Source: three-view drawing plus pictorial views. Frame: mm from the lowest corner of the part. Give positions to 0.01 mm unless a question says otherwise; leave off trailing zeros. Order: outer loops, then holes, each group sorted by start corner. A loop starts at its lowest first (then second) coordinate and runs counter-clockwise, first axis right, second up. Notation, with made-up numbers: (-35, -9.5) -> (-23, -9.5) arc R24 cw to (-23, 26.5) -> close; hole circle Ø10 at (-27, 15.25). An arc over 180 degrees is marked (long way). One line per question, with ' | ' between items.
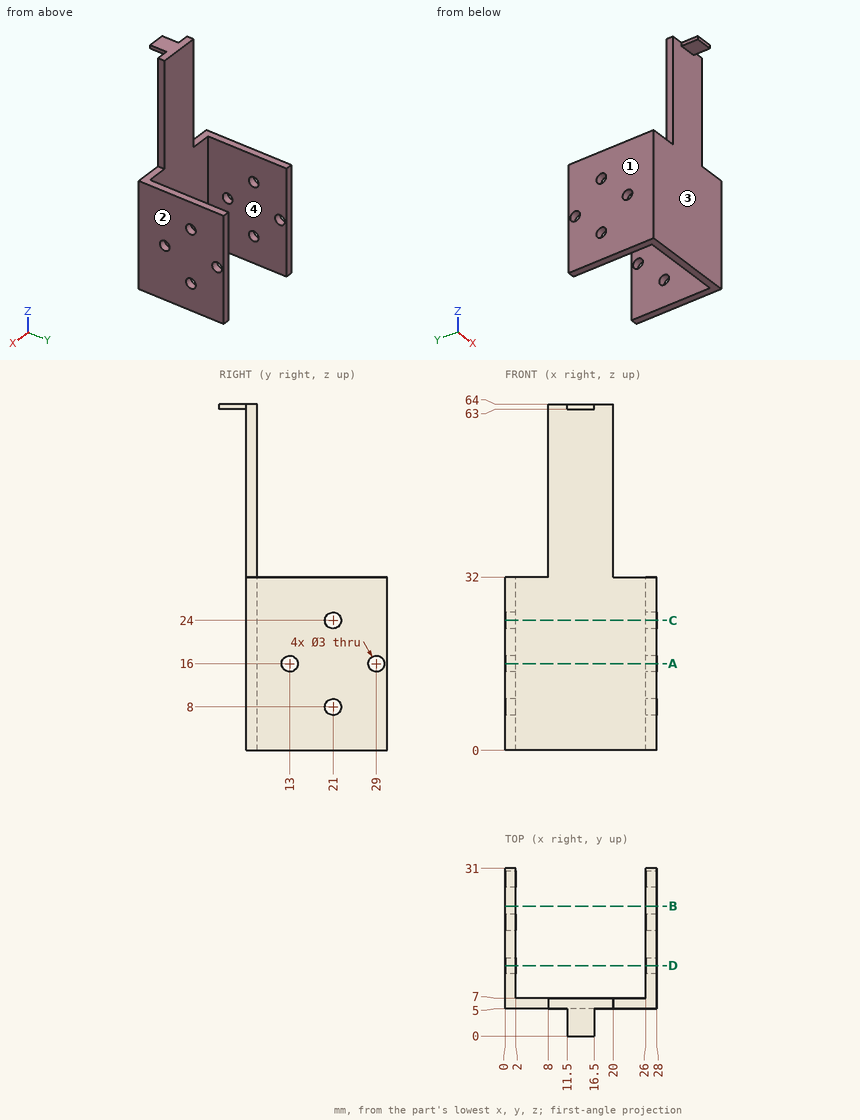
1) Pull-direction query (X, two-part tool) for the marked faces 1, 2, 3 and 4; classes: +X half, -X half, draft (parallel to the pull), parting line (faces both ways), or undercut.
Check result:
face 1: -X half | face 2: +X half | face 3: draft | face 4: undercut
2) Material intervals for probe 1 along Z at (x, y) = (0.5, 21); probe 2 along Y at (x, z) = (26.7, 16); probe 3 along X at (y, z) = (12.5, 20), sorted ascending. Write a range as from..to.
Check result:
probe 1: z = 0..6.5, 9.5..22.5, 25.5..32 | probe 2: y = 5..11.5, 14.5..27.5, 30.5..31 | probe 3: x = 0..2, 26..28
3) Section B-B on y = 24. Return loops of the section in (x, z), plus the area to 3 significant figures.
Check result:
outline: (0, 0) -> (2, 0) -> (2, 32) -> (0, 32) -> close; (26, 0) -> (28, 0) -> (28, 32) -> (26, 32) -> close | area: 128 mm^2
4) Section A-A on z = 16. Return loops of the section in (x, y), plus the area to 3 significant figures.
Check result:
outline: (0, 5) -> (28, 5) -> (28, 11.5) -> (26, 11.5) -> (26, 7) -> (2, 7) -> (2, 11.5) -> (0, 11.5) -> close; (0, 14.5) -> (2, 14.5) -> (2, 27.5) -> (0, 27.5) -> close; (0, 30.5) -> (2, 30.5) -> (2, 31) -> (0, 31) -> close; (26, 14.5) -> (28, 14.5) -> (28, 27.5) -> (26, 27.5) -> close; (26, 30.5) -> (28, 30.5) -> (28, 31) -> (26, 31) -> close | area: 128 mm^2
5) Section D-D on y = 13. Return loops of the section in (x, z).
Check result:
outline: (0, 0) -> (2, 0) -> (2, 14.5) -> (0, 14.5) -> close; (0, 17.5) -> (2, 17.5) -> (2, 32) -> (0, 32) -> close; (26, 0) -> (28, 0) -> (28, 14.5) -> (26, 14.5) -> close; (26, 17.5) -> (28, 17.5) -> (28, 32) -> (26, 32) -> close
6) Contact query for flat-ended pins moving along their axis: pin 1 Ø6 at (x, y) = (23.5, 24.5) entering from +Z; pin 2 Ø5 at (x, z) = (10, 12) entering from -Y; pin 3 Ø1.1 at (y, z) = (2, 63.5) entering from +X. Output: stop coordinate, or through.
Check result:
pin 1: stops at z = 32 | pin 2: stops at y = 5 | pin 3: stops at x = 16.5
7) Section C-C on z = 24. Return loops of the section in (x, y), plus the area to 3 significant figures.
Check result:
outline: (0, 5) -> (28, 5) -> (28, 19.5) -> (26, 19.5) -> (26, 7) -> (2, 7) -> (2, 19.5) -> (0, 19.5) -> close; (0, 22.5) -> (2, 22.5) -> (2, 31) -> (0, 31) -> close; (26, 22.5) -> (28, 22.5) -> (28, 31) -> (26, 31) -> close | area: 140 mm^2
